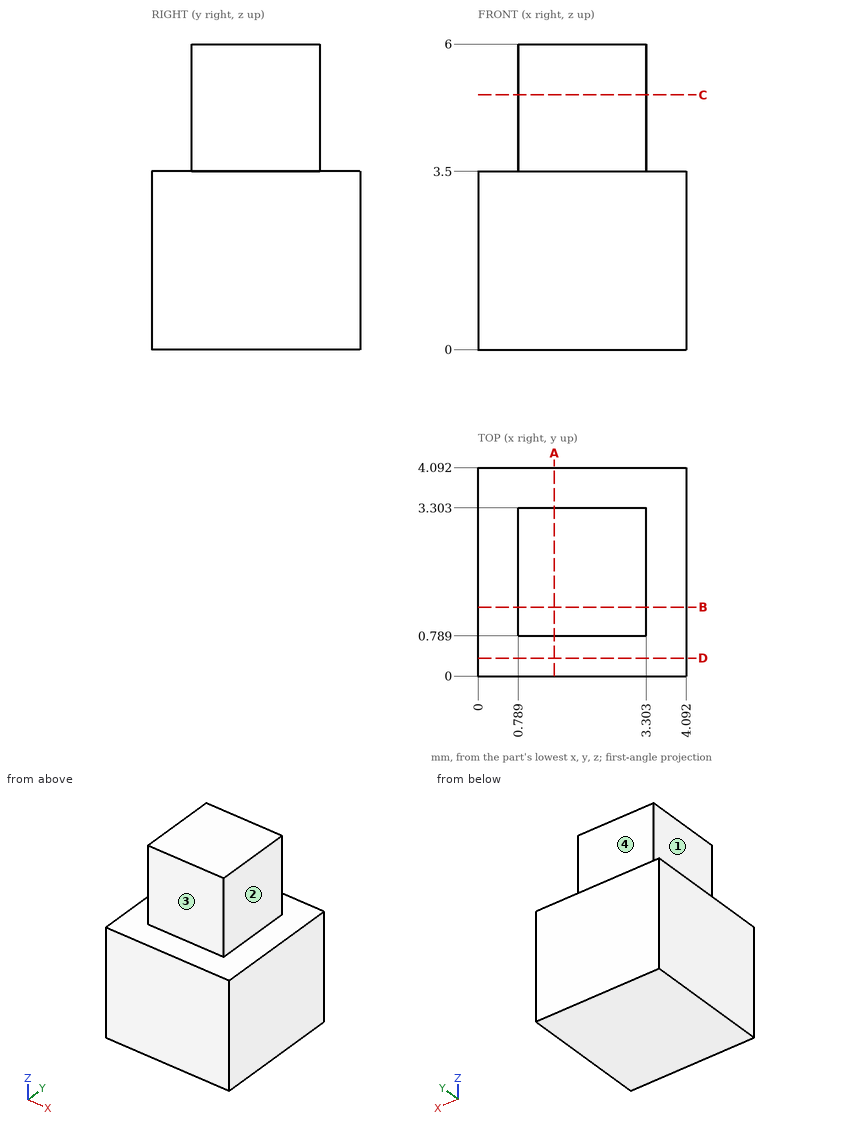
Can you work these out from the drawing? Everything is in mm from the part's minimum corner. A direction names the side the tool comes from. Give positions to 0.01 mm unless a question says otherwise; leave off trailing zeros. Loops run counter-clockwise (first coordinate to the right, second up) from the corner with the lowest first, then second, coordinate; pieces in that order, holes last. Notation, with made-up numbers: (81, 55) - (128, 55) arc R31 cw to (128, 79) - close; hole circle Ø4 at (58, 72.25). An arc over 180 degrees is marked (long way). Answer as a JSON object with one key per item and string values.
Q1. Which directions (+Z, -Z, +X, -X, +Y, -Y) give clear straight access to the entire face, cutting with the end or side of a thin tool? Please do the marked faces 1, 2, 3 and 4.
Geometry says:
{"face 1": "+Z, -X, +Y, -Y", "face 2": "+Z, +X, +Y, -Y", "face 3": "+Z, +X, -X, -Y", "face 4": "+Z, +X, -X, +Y"}
Q2. Imagine slicing it at C-C on z = 5. Write out the boundary of the cut face in (x, y), plus the area to 3 significant figures.
Geometry says:
{"outline": "(0.79, 0.79) - (3.3, 0.79) - (3.3, 3.3) - (0.79, 3.3) - close", "area": "6.32 mm²"}
Q3. Imagine slicing it at A-A on x = 1.5. Write out the boundary of the cut face in (y, z), plus the area to 3 significant figures.
Geometry says:
{"outline": "(0, 0) - (4.09, 0) - (4.09, 3.5) - (3.3, 3.5) - (3.3, 6) - (0.79, 6) - (0.79, 3.5) - (0, 3.5) - close", "area": "20.6 mm²"}
Q4. Will these pins go through, and if not, where does the flat tip stop? P1, Ø1.2, axis at y = 2, z = 5, coming from the -X side; P2, Ø0.8, axis at x = 2, z = 5, coming from the +Y side; P3, Ø0.8, axis at y = 2, z = 4.5, coming from the +X side.
Geometry says:
{"P1": "x = 0.79", "P2": "y = 3.3", "P3": "x = 3.3"}
Q5. If I drill on L1, parallel to Z at x = 1.15, y = 3.45; L2, parallel to X at y = 2.5, z = 4.35, over which ranges is the centre line in solid material (lowest first)?
Geometry says:
{"L1": "0 to 3.5", "L2": "0.79 to 3.3"}
Q6. Imagine slicing it at D-D on y = 0.35. Write out the boundary of the cut face in (x, z).
Geometry says:
{"outline": "(0, 0) - (4.09, 0) - (4.09, 3.5) - (0, 3.5) - close"}
